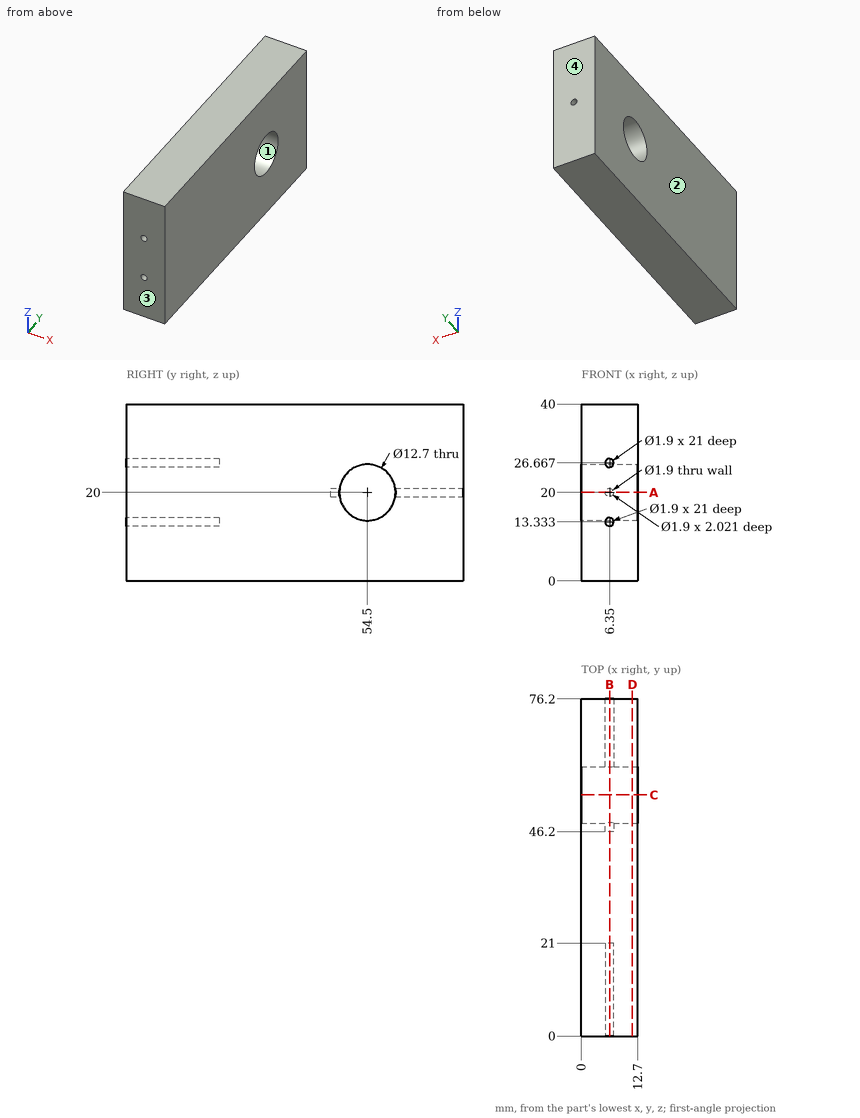
The figure shows three views and two pictorial views of one solid part (mm, origin at its lowest corner). Answer the questions. Give positions to 0.01 mm unless a question says otherwise; leave off trailing zeros. Write each loop counter-clockwise with the first axis right and the second up, starting at its lowest first coordinate (ties: lowest second). Pieces come first, ordered by that corner, then holes. Notation, with made-up numbers: (18.25, 62) - (67.25, 62) arc R18 ccw to (67.25, 94) - close; hole circle Ø1 at (13.25, 12.5). An arc over 180 degrees is marked (long way). Use CSV: the item, a comma, the result in double quotes. Start each with the question number.
Item 1: The part is cut by section B-B, the plane x = 6.35. Give the vertices of the cut face in (y, z), and give its area (3 significant figures).
Item 2: The part is cut by section C-C, the plane y = 54.5. Give the vertices of the cut face in (x, z), and give its area (3 significant figures).
Item 3: Consider line 1 (Z direction, x = 6.35, y = 12.25); line 2 (X direction, y = 72, z = 20); line 3 (Y direction, x = 9.25, z = 24.5). Determine where each line is inside the solid, lowest interval first.
Item 4: The part is cut by section A-A, the plane z = 20. Give the vertices of the cut face in (x, y).
Item 5: The part is cut by section D-D, the plane x = 11.5. Give the vertices of the cut face in (y, z), and give its area (3 significant figures).
Item 6: Flat-ended cylindrical pins translate along their axes: P1, Ø3, axis at x = 6.35, z = 20, coming from the -Y side; P2, Ø0.6, axis at x = 6, z = 13, coming from the -Y side; P3, Ø1.1, axis at x = 6.35, z = 20, coming from the +Y side. Find the tip coordinate at first contact, or state that the pin passes through.
Item 7: The mould has two halves that part along Y. Classify the marked faces 1, 2, 3 and 4: pulls with the +Y half, pulls with the -Y half, needs draft (parallel to the pull), parting line crosses it, or undercut.
Taken from the geometry:
1,outline,"(0, 0) - (76.2, 0) - (76.2, 19.05) - (60.78, 19.05) arc R6.35 cw to (48.22, 19.05) - (46.2, 19.05) - (46.2, 20.95) - (48.22, 20.95) arc R6.35 cw to (60.78, 20.95) - (76.2, 20.95) - (76.2, 40) - (0, 40) - (0, 27.62) - (21, 27.62) - (21, 25.72) - (0, 25.72) - (0, 14.28) - (21, 14.28) - (21, 12.38) - (0, 12.38) - close"
1,area,"2,810 mm2"
2,outline,"(0, 0) - (12.7, 0) - (12.7, 13.65) - (0, 13.65) - close; (0, 26.35) - (12.7, 26.35) - (12.7, 40) - (0, 40) - close"
2,area,"347 mm2"
3,line 1,"0 to 12.38, 14.28 to 25.72, 27.62 to 40"
3,line 2,"0 to 5.4, 7.3 to 12.7"
3,line 3,"0 to 50.02, 58.98 to 76.2"
4,outline,"(0, 0) - (12.7, 0) - (12.7, 48.15) - (7.3, 48.15) - (7.3, 46.2) - (5.4, 46.2) - (5.4, 48.15) - (0, 48.15) - close; (0, 60.85) - (5.4, 60.85) - (5.4, 76.2) - (0, 76.2) - close; (7.3, 60.85) - (12.7, 60.85) - (12.7, 76.2) - (7.3, 76.2) - close"
5,outline,"(0, 0) - (76.2, 0) - (76.2, 40) - (0, 40) - close; hole circle Ø12.7 at (54.5, 20)"
5,area,"2,920 mm2"
6,P1,"y = 0"
6,P2,"y = 21"
6,P3,"y = 46.2"
7,face 1,"undercut"
7,face 2,"needs draft"
7,face 3,"pulls with the -Y half"
7,face 4,"pulls with the +Y half"
